```python
from build123d import *

# Parameters (mm, degrees)
F0_W     = 287.5
F0_H     = 451
F1_DEPTH = 7
F2_R     = 30
F2_R_2   = 19.5
F3_DEPTH = 10
F4_DEPTH = 25
F5_DEPTH = 24
F2_R_3   = 17.5
F6_DEPTH = 100
F7_R     = 12
F8_DEPTH = 23


with BuildPart() as f1:
    # F0 (on Front) → F1 (new body)
    with BuildSketch(Plane.XZ):
        Rectangle(F0_W, F0_H)
    extrude(amount=F1_DEPTH)

    # F2 (on face) → F3 (join)
    with BuildSketch(Plane.XZ.offset(7)):
        with Locations((98.75, 138.5)):
            Circle(F2_R)
        with Locations((98.75, 138.5)):
            Circle(F2_R_2, mode=Mode.SUBTRACT)
    extrude(amount=F3_DEPTH)

    # F4 (cut): a face of the model
    f4_faces = [f1.faces().sort_by_distance(p)[0] for p in [
        (98.75, -7, 138.5),
    ]]
    extrude(f4_faces, amount=-F4_DEPTH, mode=Mode.SUBTRACT)

    # F5 (add): a face of the model
    f5_faces = [f1.faces().sort_by_distance(p)[0] for p in [
        (69.5985281374, -17, 138.5),
    ]]
    extrude(f5_faces, amount=-F5_DEPTH)

    # F2 (on face) → F6 (join)
    with BuildSketch(Plane.XZ.offset(7)):
        with Locations((0, -97.5)):
            Circle(F2_R_3)
    extrude(amount=F6_DEPTH)

    # F7 (on face) → F8 (join)
    with BuildSketch(Plane.XZ.offset(107)):
        with Locations((0, -97.5)):
            Circle(F7_R)
    extrude(amount=F8_DEPTH)


solid = f1.part
```
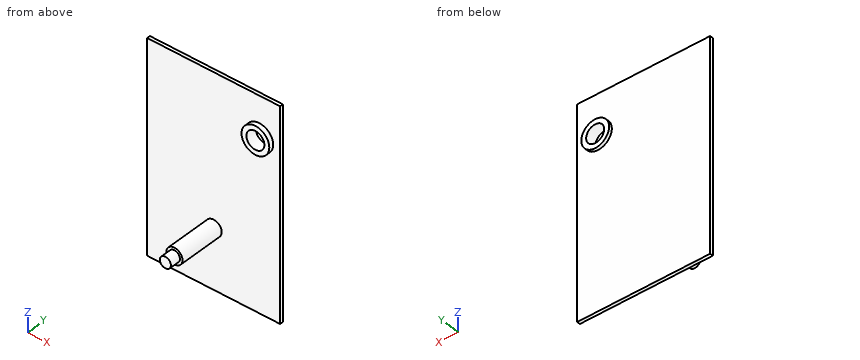
Geometry: final body of the model. Coordinates: model frame, mm. Coordinates: 2 decimals unless noted, no trailing zeros. Order: outer loops, then holes, each group sorted by start corner. A loop starts at its lowest first (then second) coordinate and runs counter-clockwise, first axis right, second up. Notation, with made-up numbers: M -11,55.5 L 20,55.5 A22 ccw 20,66.5 Z; hole C 33.5,76.25 d2. An arc over 180 degrees is marked long. Answer as CSV lines item,"result".
Q1. Section D-D on x = 0. Return the cut outline in (y, z), and give its area (3 significant figures).
Answers:
outline,"M -130,-109.5 L -107,-109.5 L -107,-115 L -7,-115 L -7,-225.5 L 0,-225.5 L 0,225.5 L -7,225.5 L -7,-80 L -107,-80 L -107,-85.5 L -130,-85.5 Z"
area,"7,210 mm^2"
Q2. Line query: probe 1 along Z at (x, y) = (98.75, -3.5); probe 2 along Z at (x, y) = (98, -10); probe 3 along Y at (x, z) = (-70, -115.5). Output: solid intervals per line, ascending. Write a range as [from, to].
Answers:
probe 1,"z = [-225.5, 119], [158, 225.5]"
probe 2,"z = [108.51, 119.01], [157.99, 168.49]"
probe 3,"y = [-7, 0]"
Q3. Section B-B on x = 98.75. Return the cut outline in (y, z), and give its area (3 significant figures).
Answers:
outline,"M -17,108.5 L -7,108.5 L -7,-225.5 L 0,-225.5 L 0,108.5 L 7,108.5 L 7,119 L -17,119 Z; M -17,158 L 7,158 L 7,168.5 L 0,168.5 L 0,225.5 L -7,225.5 L -7,168.5 L -17,168.5 Z"
area,"3,240 mm^2"
Q4. Section C-C on z = -97.5. Return the cut outline in (x, y).
Answers:
outline,"M -143.75,-7 L -17.5,-7 L -17.5,-107 L -12,-107 L -12,-130 L 12,-130 L 12,-107 L 17.5,-107 L 17.5,-7 L 143.75,-7 L 143.75,0 L -143.75,0 Z"
Q5. First-contact query: P1, Ø6, axis at x = -100, z = 11, coming from the +Y side; P2, Ø3, axis at x = -110.5, z = -137.5, coming from the -Y side; P3, Ø18, axis at x = 109.5, z = 131, coming from the -Y side. Flat tips, straight axial feed; report the tip coordinate or a pass-through.
Answers:
P1,"stops at y = 0"
P2,"stops at y = -7"
P3,"stops at y = -17"
Q6. Section A-A on z = 138.5. Return the cut outline in (x, y), and give its area (3 significant figures).
Answers:
outline,"M -143.75,-7 L 68.75,-7 L 68.75,-17 L 79.25,-17 L 79.25,7 L 68.75,7 L 68.75,0 L -143.75,0 Z; M 118.25,-17 L 128.75,-17 L 128.75,-7 L 143.75,-7 L 143.75,0 L 128.75,0 L 128.75,7 L 118.25,7 Z"
area,"2,100 mm^2"
